```python
from build123d import *

# Parameters (mm, degrees)
F1_DEPTH       = 12.6
F4_D           = 2
F4_DEPTH       = 38
F4_CBORE_D     = 3.5
F4_CBORE_DEPTH = 3
F5_D           = 2
F5_DEPTH       = 38
F5_CBORE_D     = 3.5
F5_CBORE_DEPTH = 3


with BuildPart() as f1:
    # F0 (on Front) → F1 (new body)
    with BuildSketch(Plane.XZ):
        Polygon((18.9, 6.34), (-18.9, 6.34), (-18.9, -6.34), (-13.5, -6.34), (-13.5, -1.34), (-11.5, -1.34), (-11.5, -6.34), (11.5, -6.34), (11.5, -1.34), (13.5, -1.34), (13.5, -6.34), (18.9, -6.34), align=None)
    extrude(amount=F1_DEPTH)

    # F4
    with Locations(Plane(origin=(0, 0, -6.34), x_dir=(1, 0, 0), z_dir=(0, 0, -1))):
        with Locations((0, 6.3)):
            CounterBoreHole(F4_D / 2, F4_CBORE_D / 2, F4_CBORE_DEPTH, depth=F4_DEPTH)

    # F5
    with Locations(Plane.XY.offset(6.34)):
        with Locations((-12.5, -6.3), (12.5, -6.3)):
            CounterBoreHole(F5_D / 2, F5_CBORE_D / 2, F5_CBORE_DEPTH, depth=F5_DEPTH)


solid = f1.part
```
Input: part model. Units: mm. Frame: model coordinates. A direction names the side the tool comes from. Give positions to 0.01 mm unless a question says otherwise; leave off trailing zeros. Order: outer loops, then holes, each group sorted by start corner. A loop starts at its lowest first (then second) coordinate and runs counter-clockwise, first axis right, second up. Notation, with made-up numbers: (-22.75, 62) - (-9.75, 62) arc R13 cw to (-9.75, 73) - close; hole circle Ø3 at (42, -32.5). An arc over 180 degrees is marked (long way). Put each result on its own line as item: value.
Item 1: Section query A-A, the plane z = -4.25. Return loops of the section in (x, y), then the cut area to 3 significant figures.
Found:
outline: (-18.9, -12.6) - (-13.5, -12.6) - (-13.5, 0) - (-18.9, 0) - close; (-11.5, -12.6) - (11.5, -12.6) - (11.5, 0) - (-11.5, 0) - close; (13.5, -12.6) - (18.9, -12.6) - (18.9, 0) - (13.5, 0) - close; hole circle Ø3.5 at (0, -6.3)
area: 416 mm^2
Item 2: Section query C-C, the plane z = 4.5. Return loops of the section in (x, y).
Found:
outline: (-18.9, -12.6) - (18.9, -12.6) - (18.9, 0) - (-18.9, 0) - close; hole circle Ø3.5 at (-12.5, -6.3); hole circle Ø2 at (0, -6.3); hole circle Ø3.5 at (12.5, -6.3)
Item 3: Contact query for flat-ended pins moving along their axis: pin 1 (0.6 mm diameter, centred on x = -12.5, y = -4, fed in from -Z); pin 2 (3 mm diameter, centred on x = -12.5, y = -6.3, fed in from +Z). Output: stop coordinate, or through.
Found:
pin 1: stops at z = -1.34
pin 2: stops at z = 3.34
Item 4: Section query D-D, the plane y = -11. Return loops of the section in (x, z).
Found:
outline: (-18.9, -6.34) - (-13.5, -6.34) - (-13.5, -1.34) - (-11.5, -1.34) - (-11.5, -6.34) - (11.5, -6.34) - (11.5, -1.34) - (13.5, -1.34) - (13.5, -6.34) - (18.9, -6.34) - (18.9, 6.34) - (-18.9, 6.34) - close
Item 5: Ray query, L1, parallel to X at y = -9, z = -5.25; L2, parallel to X at y = -6.3, z = -1; L3, parallel to Y at x = 12.5, z = 5.1. Return the intervals inside material, ascending. Write a range as from..to.
Found:
L1: x = -18.9..-13.5, -11.5..11.5, 13.5..18.9
L2: x = -18.9..-13.5, -11.5..-1, 1..11.5, 13.5..18.9
L3: y = -12.6..-8.05, -4.55..0
Item 6: Access query for faces 1 (the cylindrical face through (0.13, -7.29, 1.57)), 2 (the flat face through (12, -2, -1.34)), 3 (the cylindrical face through (13.31, -7.85, 4.86)), 4 (the flat face through (0, -5, 6.34)), 5 (the flat face through (0, -5, -3.34)). Directions: +Z, -Z, +X, -X, +Y, -Y. A direction counts if a zero-diameter tool reaches every point of the face in a straight line with its end or side. Return the directions, or none.
Found:
face 1: +Z, -Z
face 2: -Z, +Y, -Y
face 3: +Z
face 4: +Z, +X, -X, +Y, -Y
face 5: -Z
Item 7: Section query B-B, the plane x = 0. Return loops of the section in (y, z), then the cut area to 3 significant figures.
Found:
outline: (-12.6, -6.34) - (-8.05, -6.34) - (-8.05, -3.34) - (-7.3, -3.34) - (-7.3, 6.34) - (-12.6, 6.34) - close; (-5.3, -3.34) - (-4.55, -3.34) - (-4.55, -6.34) - (0, -6.34) - (0, 6.34) - (-5.3, 6.34) - close
area: 130 mm^2
Item 8: Draft query along X for faces 6 (the flat face through (0, 0, 0)), 7 (the cylindrical face through (13.3, -6.9, 1)). Return one class per face: +X half, -X half, draft (parallel to the pull), parting line (faces both ways), or undercut.
Found:
face 6: draft
face 7: undercut
